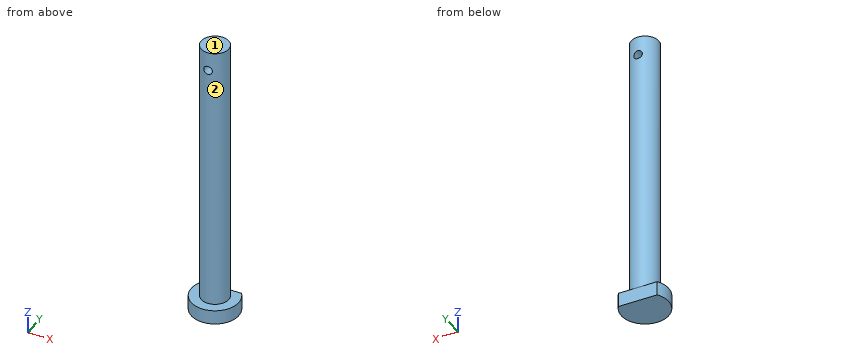
from build123d import *

# Parameters (mm, degrees)
SKETCH1_R            = 2.9
BOSS_EXTRUDE1_DEPTH  = 57
BOSS_EXTRUDE2_START  = -3
SKETCH1_3_R          = 5
SKETCH1_3_R_2        = 2.9
BOSS_EXTRUDE2_DEPTH  = 3
INTERSECT1_START     = 2.9
INTERSECT1_OUTLINE_W = 12
INTERSECT1_OUTLINE_H = 3
INTERSECT1_DEPTH     = 2.1
SKETCH2_R            = 0.9
CUT_EXTRUDE1_DEPTH   = 58.761665488


# Read off the part's stored shape, not the designer's step: Intersect1
with BuildPart() as part:
    # Sketch1 → Boss-Extrude1 (new body)
    with BuildSketch(Plane.XY):
        with Locations(Location((0, 0, 0), (0, 0, 180))):
            Circle(SKETCH1_R)
    extrude(amount=BOSS_EXTRUDE1_DEPTH)

    # Sketch1<3> → Boss-Extrude2 (add)
    # profile 1 of 2: a face of its own
    with BuildSketch(Plane.XY.offset(BOSS_EXTRUDE2_START)):
        Circle(SKETCH1_3_R)
        with Locations(Location((0, 0, 0), (0, 0, 180))):
            Circle(SKETCH1_3_R_2, mode=Mode.SUBTRACT)
    # profile 2 of 2: a face of its own
    with BuildSketch(Plane.XY.offset(BOSS_EXTRUDE2_START)):
        with Locations(Location((0, 0, 0), (0, 0, 180))):
            Circle(SKETCH1_3_R_2)
    extrude(amount=BOSS_EXTRUDE2_DEPTH)

    # Intersect1 outline → Intersect1 (cut)
    with BuildSketch(Plane(origin=(0, 0, 0), x_dir=(1, 0, 0), z_dir=(0, 1, 0)).offset(INTERSECT1_START)):
        with Locations((0, 1.5)):
            Rectangle(INTERSECT1_OUTLINE_W, INTERSECT1_OUTLINE_H)
    extrude(amount=INTERSECT1_DEPTH, mode=Mode.SUBTRACT)

    # Sketch2 → Cut-Extrude1 (cut, through all)
    with BuildSketch(Plane(origin=(0, 2.9, 0), x_dir=(1, 0, 0), z_dir=(0, 1, 0))):
        with Locations(Location((0, -53, 0), (0, 0, 270))):
            Circle(SKETCH2_R)
    extrude(amount=-CUT_EXTRUDE1_DEPTH, mode=Mode.SUBTRACT)


solid = part.part
Verification items for the finished model (mm, model axes). Face numbers are marked on the shaded views. A direction names the side the tool comes from. Give positions to 0.01 mm unless a question says otherwise; leave off trailing zeros. Order: outer loops, then holes, each group sorted by start corner. A loop starts at its lowest first (then second) coordinate and runs counter-clockwise, first axis right, second up. Notation, with made-up numbers: M 71,14 L 81,14 A12 ccw 81,35 Z; hole C 54,87.5 d11. An arc over 180 degrees is marked long. Answer as a JSON object with one key per item and string values. Group by question number.
1) Scan lines: line 1 along Z through (x, y) = (0, 1.1); line 2 along Z through (x, y) = (3.5, 0.5); line 3 along Y through (x, z) = (-0.25, 26.5). Record each from-to range of solid material in increasing order. Write a range as [from, to].
2) Cross-section at B-B (z = 41). Enter the section's corners in (x, y), then the cut area to 3 significant figures.
3) Access from +Z, -Z, +X, -X, +Y, -Y to the whole of each face (thin tool, end or side, straight path). Record for the marked faces 1 and 2.
4) Cross-section at A-A (y = 0). Enter the section's corners in (x, z).
5) Cross-section at D-D (y = -3.5). Enter the section's corners in (x, z), then the cut area to 3 significant figures.
6) Depth check by flat-ended pin: pin 1 Ø3 at (y, z) = (0, 9.5) entering from +X; pin 2 Ø3 at (x, z) = (-1.5, 49) entering from -Y; pin 3 Ø1.5 at (x, z) = (2.5, 19) entering from -Y. Enter the tip coordinate at first touch or a pass-through.
7) Cross-section at C-C (x = 1.75). Enter the section's corners in (y, z).
Result sheet:
{
 "1": {"line 1": "z = [-3, 52.1], [53.9, 57]", "line 2": "z = [-3, 0]", "line 3": "y = [-2.89, 2.89]"},
 "2": {"outline": "C 0,0 d5.8", "area": "26.4 mm2"},
 "3": {"face 1": "+Z, +X, -X, +Y, -Y", "face 2": "+Z"},
 "4": {"outline": "M -5,-3 L 5,-3 L 5,0 L 2.9,0 L 2.9,57 L -2.9,57 L -2.9,0 L -5,0 Z; hole C 0,53 d1.8"},
 "5": {"outline": "M -3.57,-3 L 3.57,-3 L 3.57,0 L -3.57,0 Z", "area": "21.4 mm2"},
 "6": {"pin 1": "stops at x = 2.9", "pin 2": "stops at y = -2.9", "pin 3": "stops at y = -2.31"},
 "7": {"outline": "M -4.68,-3 L 2.9,-3 L 2.9,0 L 2.31,0 L 2.31,57 L -2.31,57 L -2.31,0 L -4.68,0 Z"}
}
